Input: part model. Units: mm. Frame: model coordinates. Face numbers are marked on the shaded views. A direction names the side the tool comes from. Give positions to 0.01 mm unless a question says otherwise; leave off trailing zeros. Loops run counter-clockwise (first coordinate to the right, second up) from the corner with the lowest first, then second, coordinate; pieces in that order, holes last. Notation, with made-up numbers: (77, 50.25) -> (93, 50.25) arc R13 ccw to (93, 73.25) -> close; hole circle Ø2 at (21.25, 67). An arc over 180 degrees is marked (long way). Answer as a JSON object with one key per item and string values.
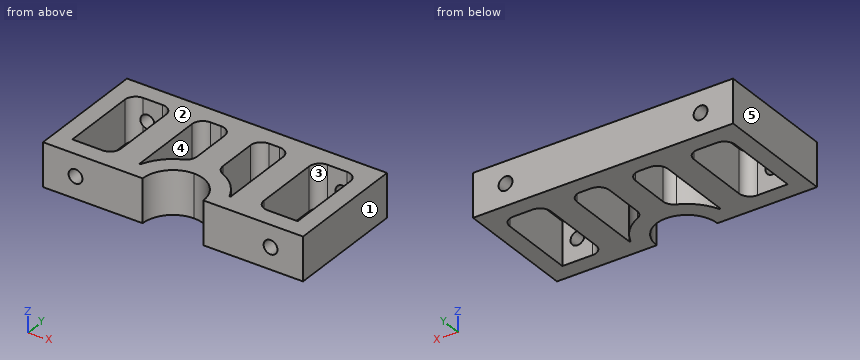
```python
from build123d import *

# Parameters (mm, degrees)
EXTRUDE_1_DEPTH     = 10
SKETCH_2_W          = 9.5
SKETCH_2_H          = 20
CUT_EXTRUDE_2_DEPTH = 15
FILLET_1_R          = 2.5
SKETCH_3_R          = 1.6
CUT_EXTRUDE_1_DEPTH = 43.237424164


with BuildPart() as part:
    # ｽｹｯﾁ1 → ﾎﾞｽ - 押し出し1 (new body)
    with BuildSketch(Plane.XY):
        with BuildLine():
            Line((-30, 28), (-30, 0))
            Line((-30, 0), (-7, 0))
            ThreePointArc((-7, 0), (-4.949747468, 4.949747468), (0, 7))
            Line((0, 7), (0, 28))
            Line((0, 28), (-30, 28))
        make_face()
        with BuildLine():
            Line((7, 0), (30, 0))
            Line((30, 0), (30, 28))
            Line((30, 28), (0, 28))
            Line((0, 28), (0, 7))
            ThreePointArc((0, 7), (4.949747468, 4.949747468), (7, 0))
        make_face()
    extrude(amount=EXTRUDE_1_DEPTH)

    # ｽｹｯﾁ2 → ｶｯﾄ - 押し出し2 (cut)
    with BuildSketch(Plane.XY.offset(10)):
        with BuildLine():
            Line((10.5, 24), (3, 24))
            Line((3, 24), (3, 10.583005244))
            ThreePointArc((3, 10.583005244), (7.396243348, 8.14221004), (10.246950766, 4))
            Line((10.246950766, 4), (10.5, 4))
            Line((10.5, 4), (10.5, 24))
        make_face()
        with BuildLine():
            Line((-3, 10.583005244), (-3, 24))
            Line((-3, 24), (-10.5, 24))
            Line((-10.5, 24), (-10.5, 4))
            Line((-10.5, 4), (-10.246950766, 4))
            ThreePointArc((-10.246950766, 4), (-7.396243348, 8.14221004), (-3, 10.583005244))
        make_face()
        with Locations((21.25, 14)):
            Rectangle(SKETCH_2_W, SKETCH_2_H)
        with Locations((-21.25, 14)):
            Rectangle(SKETCH_2_W, SKETCH_2_H)
    extrude(amount=-CUT_EXTRUDE_2_DEPTH, mode=Mode.SUBTRACT)

    # ﾌｨﾚｯﾄ1
    fillet_1_edges = [part.edges().sort_by_distance(p)[0] for p in [
        (16.5, 4, 5),
        (16.5, 24, 5),
        (26, 24, 5),
        (3, 10.583005244, 5),
        (3, 24, 5),
        (10.5, 24, 5),
        (-3, 10.583005244, 5),
        (-10.5, 24, 5),
        (-3, 24, 5),
        (-16.5, 4, 5),
        (-26, 24, 5),
        (-16.5, 24, 5),
    ]]
    fillet(fillet_1_edges, radius=FILLET_1_R)

    # ｽｹｯﾁ3 → ｶｯﾄ - 押し出し1 (cut, through all)
    with BuildSketch(Plane(origin=(0, 28, 0), x_dir=(1, 0, 0), z_dir=(0, 1, 0))):
        with Locations(Location((-22.5, -5, 0), (0, 0, 270))):
            Circle(SKETCH_3_R)
        with Locations(Location((22.5, -5, 0), (0, 0, 270))):
            Circle(SKETCH_3_R)
    extrude(amount=-CUT_EXTRUDE_1_DEPTH, mode=Mode.SUBTRACT)


solid = part.part
```
Q1. Section A-A, the plane x = -22.5. Return the cut outline in (y, z).
Evaluation:
{"outline": "(0, 0) -> (4, 0) -> (4, 3.4) -> (0, 3.4) -> close; (0, 6.6) -> (4, 6.6) -> (4, 10) -> (0, 10) -> close; (24, 0) -> (28, 0) -> (28, 3.4) -> (24, 3.4) -> close; (24, 6.6) -> (28, 6.6) -> (28, 10) -> (24, 10) -> close"}
Q2. Section D-D, the plane z = 5. Give the number of separate pieces and of enclosed holes in the cut face, then the cut area to 3 significant figures.
Evaluation:
{"separate pieces": "3", "enclosed holes": "2", "area": "949 mm2"}
Q3. Ray query, line 1 along X through (y, z) = (27, 5); line 2 along X through (y, z) = (21.25, 8); line 3 along X through (y, z) = (1.3, 5). Return the intervals inside material, ascending.
Evaluation:
{"line 1": "x = -30 to -24.1, -20.9 to 20.9, 24.1 to 30", "line 2": "x = -30 to -26, -16.5 to -10.5, -3 to 3, 10.5 to 16.5, 26 to 30", "line 3": "x = -30 to -24.1, -20.9 to -6.88, 6.88 to 20.9, 24.1 to 30"}
Q4. Section C-C, the plane x = -9. Return the cut outline in (y, z), then the cut area to 3 significant figures.
Evaluation:
{"outline": "(0, 0) -> (6.32, 0) -> (6.32, 10) -> (0, 10) -> close; (23.79, 0) -> (28, 0) -> (28, 10) -> (23.79, 10) -> close", "area": "105 mm2"}
Q5. Section B-B, the plane y = 17.75. Return the cut outline in (x, z).
Evaluation:
{"outline": "(-30, 0) -> (-26, 0) -> (-26, 10) -> (-30, 10) -> close; (-16.5, 0) -> (-10.5, 0) -> (-10.5, 10) -> (-16.5, 10) -> close; (-3, 0) -> (3, 0) -> (3, 10) -> (-3, 10) -> close; (10.5, 0) -> (16.5, 0) -> (16.5, 10) -> (10.5, 10) -> close; (26, 0) -> (30, 0) -> (30, 10) -> (26, 10) -> close"}
Q6. Draft query along X for the marked faces 1, 2 and 3. Return one class per face: +X half, -X half, draft (parallel to the pull), parting line (faces both ways), or undercut.
Evaluation:
{"face 1": "+X half", "face 2": "draft", "face 3": "undercut"}
Q7. Pin query (flat end, axial travel): pin 1 (3 mm diameter, centred on x = 3, y = 14, fed in from -Z); pin 2 (1.9 mm diameter, centred on x = 22.5, z = 5, fed in from +Y). Return the tip coordinate at first contact, or that it passes through.
Evaluation:
{"pin 1": "stops at z = 0", "pin 2": "passes through"}
Q8. Access query for the marked faces 4 and 5. Directions: +Z, -Z, +X, -X, +Y, -Y. A direction counts if a zero-diameter tool reaches every point of the face in a straight line with its end or side. Return the directions, or none.
Evaluation:
{"face 4": "+Z, -Z", "face 5": "+Z, -Z, -X, +Y, -Y"}
